from build123d import *

# Parameters (mm, degrees)
SKETCH2_R           = 14.75
BOSS_EXTRUDE1_DEPTH = 7.5
BOSS_EXTRUDE2_START = -7.5
SKETCH3_R           = 20
BOSS_EXTRUDE2_DEPTH = 1
SKETCH4_R           = 12.5
CUT_EXTRUDE1_DEPTH  = 10


with BuildPart() as part:
    # Sketch2 → Boss-Extrude1 (new body, symmetric)
    with BuildSketch(Plane.XY):
        Circle(SKETCH2_R)
    extrude(amount=BOSS_EXTRUDE1_DEPTH, both=True)

    # Sketch3 → Boss-Extrude2 (add)
    with BuildSketch(Plane.XY.offset(BOSS_EXTRUDE2_START)):
        Circle(SKETCH3_R)
    extrude(amount=BOSS_EXTRUDE2_DEPTH)

    # Sketch4 → Cut-Extrude1 (cut)
    with BuildSketch(Plane(origin=(0, 0, -7.5), x_dir=(-1, 0, 0), z_dir=(0, 0, -1))):
        Circle(SKETCH4_R)
    extrude(amount=-CUT_EXTRUDE1_DEPTH, mode=Mode.SUBTRACT)


solid = part.part
Part model, mm, in its own coordinate system. A direction names the side the tool comes from. Coordinates: 2 decimals unless noted, no trailing zeros. Loops run counter-clockwise (first coordinate to the right, second up) from the corner with the lowest first, then second, coordinate; pieces in that order, holes last. Notation, with made-up numbers: (34, 74) -> (47, 74) arc R33 ccw to (47, 110) -> close; hole circle Ø6 at (65, 39). An arc over 180 degrees is marked (long way). Use a Markdown table: item, result. Add a question column.
Item 1: Pull direction Y, two halves, no side cores. Call faces 1 (the flat face through (0, 0, 7.5)), 2 (the cylindrical face through (-4.336, -19.524, -7.007)), 3 (the cylindrical face through (-11.923, 3.755, -2.57)): +Y half, -Y half, draft (parallel to the pull), parting line (faces both ways), or undercut.
Item 2: Band-saw the part on C-C on z = -1.5. Write the cut outline in (x, y).
Item 3: Probe probe 1 along Y at (x, z) = (0, -3); probe 2 along X at (y, z) = (0.5, 2); probe 3 along Y at (x, z) = (-10, -2.5). List the from-to ranges inside material, lowest first.
Item 4: Band-saw the part on A-A on x = 0. Write the cut outline in (y, z), plus the area to 3 significant figures.
Item 5: Band-saw the part on D-D on z = 5.5. Write the cut outline in (x, y).
Item 6: Which spindle directions (+Z, -Z, +X, -X, +Y, -Y) get a long thin tool onto all of the face, cutting with end or side? Do faces 4 (the flat face through (-2, -15, -6.5)), 5 (the flat face through (0, 0, 2.5)), 6 (the flat face through (9, 9, -7.5)). Say none if no direction does.
Item 7: Flat gauge pins, fed straight in: P1, Ø2, axis at y = -13, z = 4, coming from the -X side; P2, Ø1.5, axis at x = 9, y = -14, coming from the +Z side; P3, Ø6, axis at x = 13, y = -12, coming from the +Z side; P4, Ø4, axis at x = -11, z = -2, coming from the +Y side. Where does each tip first touch, or does it go through?
Geometry says:
| question | item | result |
|---|---|---|
| 1 | face 1 | draft |
| 1 | face 2 | parting line |
| 1 | face 3 | undercut |
| 2 | outline | circle Ø29.5 at (0, 0); hole circle Ø25 at (0, 0) |
| 3 | probe 1 | -14.75 to -12.5, 12.5 to 14.75 |
| 3 | probe 2 | -14.74 to -12.49, 12.49 to 14.74 |
| 3 | probe 3 | -10.84 to -7.5, 7.5 to 10.84 |
| 4 | outline | (-20, -7.5) -> (-12.5, -7.5) -> (-12.5, 2.5) -> (12.5, 2.5) -> (12.5, -7.5) -> (20, -7.5) -> (20, -6.5) -> (14.75, -6.5) -> (14.75, 7.5) -> (-14.75, 7.5) -> (-14.75, -6.5) -> (-20, -6.5) -> close |
| 4 | area | 203 mm² |
| 5 | outline | circle Ø29.5 at (0, 0) |
| 6 | face 4 | +Z |
| 6 | face 5 | -Z |
| 6 | face 6 | -Z, +X, -X, +Y, -Y |
| 7 | P1 | x = -8.58 |
| 7 | P2 | z = -6.5 |
| 7 | P3 | z = 7.5 |
| 7 | P4 | y = 11.69 |
